Geometry check sheet. Reference: the model listing, model coordinates, mm. A direction names the side the tool comes from. Round coordinates to 2 decimals unless told otherwise and drop trailing zeros. Order: outer loops, then holes, each group sorted by start corner. A loop starts at its lowest first (then second) coordinate and runs counter-clockwise, first axis right, second up.
```python
from build123d import *

# Parameters (mm, degrees)
SKETCH1_W          = 843
SKETCH1_H          = 960
BASE_FLANGE1_DEPTH = 1.5


# Sheet-metal steps are written as plain solids
with BuildPart() as part:
    # Sketch1 → Base-Flange1 (new body)
    with BuildSketch(Plane.XY):
        with Locations((0, 480)):
            Rectangle(SKETCH1_W, SKETCH1_H)
        Polygon((-340, 500), (-340, 103.5), (-296.5, 60), (296.5, 60), (340, 103.5), (340, 500), align=None, mode=Mode.SUBTRACT)
    extrude(amount=-BASE_FLANGE1_DEPTH)


solid = part.part
```
(1) Sectioned sample at B-B, the plane y = 331.5. Record the cut outline in (x, z), and give its area (4 significant figures).
Returned:
outline: (-421.5, -1.5) - (-340, -1.5) - (-340, 0) - (-421.5, 0) - close; (340, -1.5) - (421.5, -1.5) - (421.5, 0) - (340, 0) - close
area: 244.5 mm2
(2) Material ranges on line 1 (Y direction, x = -74, z = -1.3); line 2 (X direction, y = 297.5, z = -0.9); line 3 (Y direction, x = -314.5, z = -0.3), recorded low to high.
Returned:
line 1: y = 0 to 60, 500 to 960
line 2: x = -421.5 to -340, 340 to 421.5
line 3: y = 0 to 78, 500 to 960
(3) Draft check along X on faces 1 (the flat face through (-318.6, 82.1, -0.7)), 2 (the flat face through (-6, 700, -1.5)). Enter one of: released by +X, released by -X, zero draft, split by the parting line, or undercut.
Returned:
face 1: undercut
face 2: zero draft
(4) Set-up check for faces 3 (the flat face through (-6, 700, 0)), 4 (the flat face through (317.9, 81.4, -0.7)): record each of +Z, -Z, +X, -X, +Y, -Y from which the full face is reachable in a straight line by a thin tool's end or side.
Returned:
face 3: +Z, +X, -X, +Y, -Y
face 4: +Z, -Z
(5) Sectioned sample at C-C, the plane x = -140.5. Record the cut outline in (y, z).
Returned:
outline: (0, -1.5) - (60, -1.5) - (60, 0) - (0, 0) - close; (500, -1.5) - (960, -1.5) - (960, 0) - (500, 0) - close
(6) Sectioned sample at A-A, the plane z = -1.2. Record the cut outline in (x, y), and give its area (3 significant figures).
Returned:
outline: (-421.5, 0) - (421.5, 0) - (421.5, 960) - (-421.5, 960) - close; hole (-340, 103.5) - (-296.5, 60) - (296.5, 60) - (340, 103.5) - (340, 500) - (-340, 500) - close
area: 512,000 mm2
